```python
from build123d import *

# Parameters (mm, degrees)
F0_W      = 14
F0_H      = 8
F0_W_2    = 10
F0_H_2    = 4
F1_DEPTH  = 16
F2_W      = 24
F2_H      = 18
F2_W_2    = 14
F2_H_2    = 8
F3_DEPTH  = 1
F4_R      = 1
F5_DEPTH  = 18.001
F6_SIZE   = 7
F9_DEPTH  = 5
F10_DEPTH = 5


with BuildPart() as f1:
    # F0 (on Top) → F1 (new body)
    with BuildSketch(Plane.XY):
        Rectangle(F0_W, F0_H)
        Rectangle(F0_W_2, F0_H_2, mode=Mode.SUBTRACT)
    extrude(amount=-F1_DEPTH)

    # F4 (on face) → F5 (cut, through all)
    with BuildSketch(Plane(origin=(0, 9, 0), x_dir=(-1, 0, 0), z_dir=(0, 1, 0))):
        with BuildLine():
            ThreePointArc((1, -28), (0, -27), (-1, -28))
            Line((-1, -28), (1, -28))
        make_face()
        with BuildLine():
            Line((1, -28), (-1, -28))
            ThreePointArc((-1, -28), (0, -29), (1, -28))
        make_face()
        with Locations((0, -4.0714931674)):
            Circle(F4_R)
    extrude(amount=-F5_DEPTH, mode=Mode.SUBTRACT)


with BuildPart() as f3:
    # F2 (on face) → F3 (new body)
    with BuildSketch(Plane.XY):
        Rectangle(F2_W, F2_H)
        Rectangle(F2_W_2, F2_H_2, mode=Mode.SUBTRACT)
    extrude(amount=-F3_DEPTH)

    # F6
    f6_edges = [f3.edges().sort_by_distance(p)[0] for p in [
        (-12, -9, -0.5),
    ]]
    chamfer(f6_edges, length=F6_SIZE)


with BuildPart() as f7_1:
    # F7: instance of F3
    add(f3.part.mirror(Plane(origin=(0, 0, -16), x_dir=(1, 0, 0), z_dir=(0, 0, -1))))


with BuildPart() as f7_2:
    # F7: instance of F1
    add(f1.part.mirror(Plane(origin=(0, 0, -16), x_dir=(1, 0, 0), z_dir=(0, 0, -1))))


with BuildPart() as f7_2_1:
    # F8: moved
    add(f7_2.part.moved(Location((0, 5, 0))))


with BuildPart() as f7_1_1:
    # F8: moved
    add(f7_1.part.moved(Location((0, 5, 0))))


with BuildPart() as f1_1:
    add(f1.part)

    # F9 (add, through all): a face of the model
    f9_faces = [f7_2_1.part.faces().sort_by_distance(p)[0] for p in [
        (0, 1, -23.9441190926),
    ]]

    add(f7_1_1.part)  # F9 merges F7_1

    add(f7_2_1.part)  # F9 merges F7_2
    extrude(f9_faces, amount=F9_DEPTH)

    # F10 (add, through all): a face of the model
    f10_faces = [f1_1.faces().sort_by_distance(p)[0] for p in [
        (0, 4, -8.0558809074),
    ]]

    add(f3.part)  # F10 merges F3
    extrude(f10_faces, amount=F10_DEPTH)


solid = f1_1.part
```
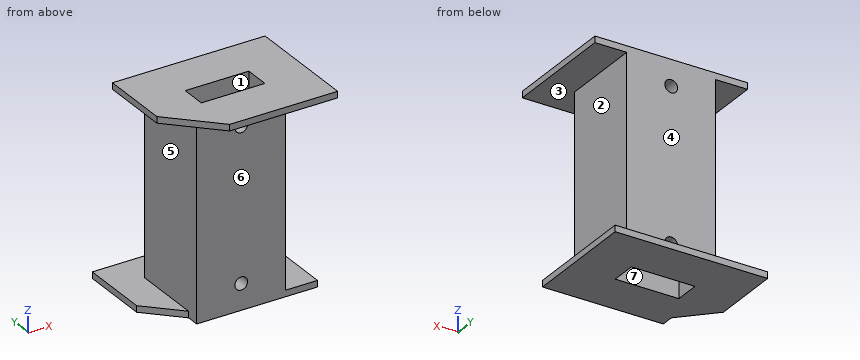
The listing builds one solid part. Answer for the finished solid, in the listing's coordinates (mm). Face numbers are marked on the shaded views. A direction names the side the tool comes from. Give positions to 0.01 mm unless a question says otherwise; leave off trailing zeros. Order: outer loops, then holes, each group sorted by start corner. A loop starts at its lowest first (then second) coordinate and runs counter-clockwise, first axis right, second up. Notation, with made-up numbers: (-29.75, -35.75) -> (26.25, -35.75) arc R34 ccw to (26.25, -3.75) -> close; hole circle Ø2 at (-4, 39). An arc over 180 degrees is marked (long way). One line per item, written item: value.
1) Find section A-A, the plane x = 0. Count the separate pieces of the cut face and the enclosed holes in it, plus the area to 3 significant figures.
Reported:
separate pieces: 5
enclosed holes: 0
area: 262 mm^2
2) Find section D-D, the plane x = -3.5. Determine the outline of the cut face in (y, z), plus the area to 3 significant figures.
Reported:
outline: (-9, -1) -> (-4, -1) -> (-4, -32) -> (3, -32) -> (3, -16) -> (7, -16) -> (7, -32) -> (14, -32) -> (14, -31) -> (9, -31) -> (9, 0) -> (2, 0) -> (2, -16) -> (-2, -16) -> (-2, 0) -> (-9, 0) -> close
area: 298 mm^2
3) Flat-ended cylindrical pins translate along their axes: P1, Ø1.8, axis at x = 0, z = -27.93, coming from the +Y side; P2, Ø2, axis at x = -5, z = -4, coming from the -Y side; P3, Ø1.5, axis at y = 2.5, z = -14.5, coming from the -X side; P4, Ø1.2, axis at x = -1.5, y = -0.5, coming from the +Z side. Find the tip coordinate at first contact, or state that the pin passes through.
Reported:
P1: passes through
P2: stops at y = -4
P3: stops at x = -7
P4: stops at z = -16
4) A tool of negligible diameter and unlimited length cuts with its end or side. For the marked faces 1, 2, 3 and 4, from which of +Z, -Z, +X, -X, +Y, -Y can it reach the whole face along a straight path? Write none if from no direction.
Reported:
face 1: +Z
face 2: +X, +Y, -Y
face 3: -Y
face 4: +Z, +X, -X, +Y
5) Find section C-C, the plane y = 1.5. Determine the outline of the cut face in (x, z).
Reported:
outline: (-12, -1) -> (-7, -1) -> (-7, -31) -> (-10.5, -31) -> (-10.5, -32) -> (12, -32) -> (12, -31) -> (7, -31) -> (7, -1) -> (12, -1) -> (12, 0) -> (5, 0) -> (5, -16) -> (-5, -16) -> (-5, 0) -> (-12, 0) -> close; hole circle Ø2 at (0, -27.93)
6) Determine the mould class of the marked faces 5, 6 and 7 for opening direction X: pulls with the +X half, pulls with the -X half, needs draft (parallel to the pull), parting line crosses it, or undercut.
Reported:
face 5: pulls with the -X half
face 6: needs draft
face 7: undercut
7) Find section B-B, the plane z = -16.5. Determine the outline of the cut face in (x, y), plus the area to 3 significant figures.
Reported:
outline: (-7, -4) -> (7, -4) -> (7, 9) -> (-7, 9) -> close; hole (-5, 3) -> (5, 3) -> (5, 7) -> (-5, 7) -> close
area: 142 mm^2
8) Find the intervals of material crossed by line 1 (Z direction, x = 0, y = -2.9); line 2 (Y direction, x = 3, z = -5.5); line 3 (Z direction, x = 0, y = 0.5), in increasing order.
Reported:
line 1: z = -32 to -28.93, -26.93 to -5.07, -3.07 to 0
line 2: y = -4 to -2, 2 to 9
line 3: z = -32 to -28.93, -26.93 to -16
